from build123d import *

# Parameters (mm, degrees)
PATTERN_CIRCULAR_1_COUNT = 4


with BuildPart() as part:
    # 草图1 → 旋转1 (revolve)
    with BuildSketch(Plane(origin=(0, 0, 0), x_dir=(0, 0, -1), z_dir=(1, 0, 0)), mode=Mode.PRIVATE) as revolve_1_sk:
        with BuildLine():
            Line((60, 0), (42.679491924, 10))
            Line((42.679491924, 10), (36.32612495, 10))
            Line((36.32612495, 10), (36.32612495, 6.632164181))
            ThreePointArc((36.32612495, 6.632164181), (18.463294368, 1.671632263), (0, 0))
            Line((0, 0), (0, -5.085825136))
            Line((0, -5.085825136), (45.191092466, -5.085825136))
            Line((45.191092466, -5.085825136), (54, 0))
            Line((54, 0), (60, 0))
        make_face()
    revolve(revolve_1_sk.sketch.rotate(Axis((0, 23.869545483, 0), (0, -1, 0)), 180), axis=Axis((0, 23.869545483, 0), (0, -1, 0)))

    # 草图2 → 切除-旋转1 (revolve, cut)
    with BuildSketch(Plane.XY, mode=Mode.PRIVATE) as cut_revolve_1_sk:
        Polygon((23.11658969, 18.792484499), (29.364790714, 20.584127312), (39.564082896, -14.98503156), (33.315881872, -16.776674373), align=None)
    cut_revolve_1 = revolve(cut_revolve_1_sk.sketch.rotate(Axis((0, 99.409613277, 0), (0.2756373558169999, -0.9612616959383187, 0)), 180), axis=Axis((0, 99.409613277, 0), (0.2756373558169999, -0.9612616959383187, 0)), mode=Mode.SUBTRACT)

    # 阵列(圆周)1: 切除-旋转1 ×4 about axis
    pattern_circular_1_axis = Axis((0, 6.632164181, 0), (0, 1, 0))
    for i in range(1, PATTERN_CIRCULAR_1_COUNT):
        add(cut_revolve_1.rotate(pattern_circular_1_axis, i * 360 / PATTERN_CIRCULAR_1_COUNT), mode=Mode.SUBTRACT)


solid = part.part
Read the model definition and answer for the solid it produces. Units are mm, in the model's axes. A direction names the side the tool comes from. Round coordinates to 2 decimals unless told otherwise and drop trailing zeros. Write each loop counter-clockwise with the first axis right and the second up, starting at its lowest first coordinate (ties: lowest second). Pieces come first, ordered by that corner, then holes.
1. Determine the mould class of faces 4 (the face through (0.286, 1.444, 34.847)), 5 (the face through (-1, -5.086, 1)), 6 (the face through (38.61, 9.514, 20.082)) for opening direction Z: pulls with the +Z half, pulls with the -Z half, needs draft (parallel to the pull), parting line crosses it, or undercut.
2. The part is cut by section A-A, the plane x = 0. Determine the outline of the cut face in (y, z).
3. Straight lines are drawn through the part: L1, parallel to Z at x = -32, y = 0.25; L2, parallel to X at y = 3, z = -30; L3, parallel to Z at x = -6, y = 7.75. For each, find the intervals that lie inside material, in ascending order.
4. The part is cut by section B-B, the plane z = 0. Determine the outline of the cut face in (x, y), then the cut area to 3 significant figures.
5. Which of the six approach directions +Z, -Z, +X, -X, +Y, -Y give full straight-line access (tool end or side, diameter ignored) to faces 1 (the face through (22.1, 8.29, -28.83)), 2 (the face through (-9, 0, 54)), 3 (the face through (34.847, 1.444, -0.286))?
6. Given pin 1 Ø1 at (x, z) = (-44, -3) entering from +Y; pin 2 Ø4 at (x, z) = (23.5, 18) entering from +Y; pin 3 Ø8 at (x, y) = (-43, 3.5) entering from +Z; pin 4 Ø3 at (x, z) = (1, -25.5) entering from -Y, each flat-ended and moving along its own axis, determine where each tip first touches the part or whether it passes through.
7. The part is cut by section C-C, the plane y = -3.5. State how many separate pieces and enclosed holes the cut face has, then the cut area to 3 significant figures.
Values:
1. face 4: undercut
1. face 5: needs draft
1. face 6: parting line crosses it
2. outline: (-5.09, -45.19) - (0, -54) - (0, -60) - (10, -42.68) - (10, -36.33) - (6.63, -36.33) arc R102.8 cw to (5.66, -33.64) - (-5.09, -36.73) - close; (-5.09, -23.2) - (2.19, -21.11) arc R102.8 cw to (2.19, 21.11) - (-5.09, 23.2) - close; (-5.09, 36.73) - (5.66, 33.64) arc R102.8 cw to (6.63, 36.33) - (10, 36.33) - (10, 42.68) - (0, 60) - (0, 54) - (-5.09, 45.19) - close
3. L1: z = -50.24 to -5.52, 5.52 to 50.24
3. L2: x = -45.86 to -6.09, 6.09 to 45.86
3. L3: z = -46.19 to -35.83, 35.83 to 46.19
4. outline: (-60, 0) - (-54, 0) - (-45.19, -5.09) - (-36.73, -5.09) - (-33.64, 5.66) arc R102.8 cw to (-36.33, 6.63) - (-36.33, 10) - (-42.68, 10) - close; (-23.2, -5.09) - (23.2, -5.09) - (21.11, 2.19) arc R102.8 cw to (-21.11, 2.19) - close; (33.64, 5.66) - (36.73, -5.09) - (45.19, -5.09) - (54, 0) - (60, 0) - (42.68, 10) - (36.33, 10) - (36.33, 6.63) arc R102.8 cw to start
4. area: 723 mm2
5. face 1: +Y
5. face 2: -Y
5. face 3: none
6. pin 1: stops at y = 9.47
6. pin 2: stops at y = 4.98
6. pin 3: stops at z = 43.75
6. pin 4: passes through
7. separate pieces: 1
7. enclosed holes: 4
7. area: 6,670 mm2
